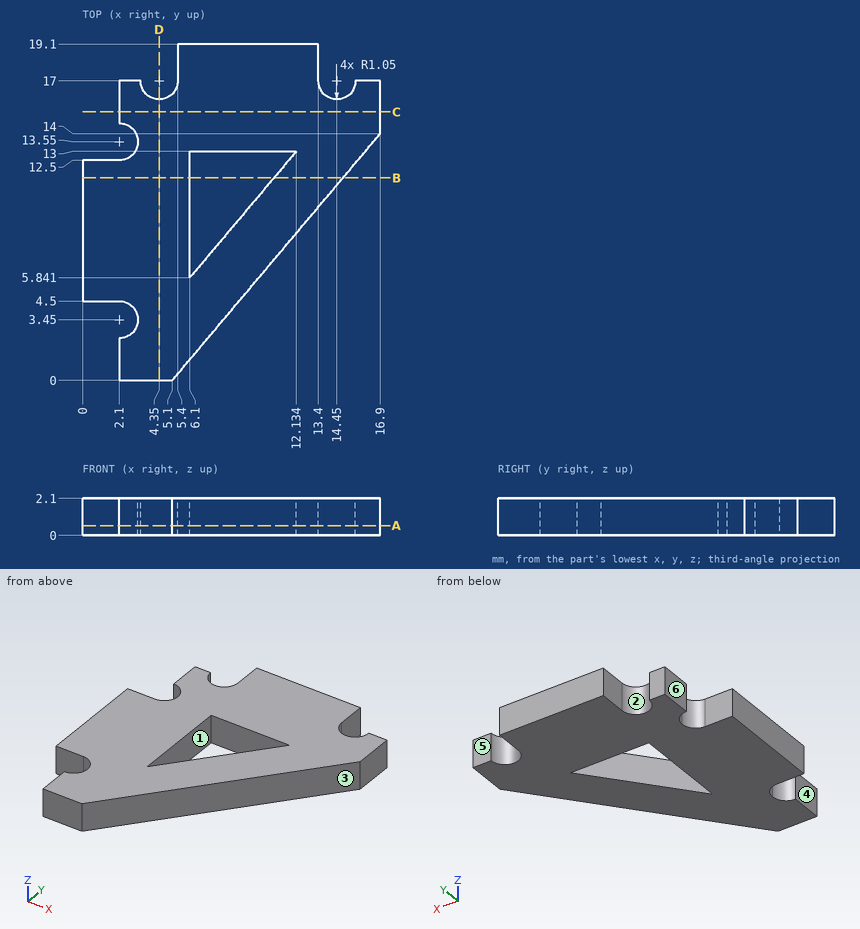
Verification items for this drawing (mm, ordinates from the low corner). A direction names the side the tool comes from. Round coordinates to 2 decimals unless told otherwise and drop trailing zeros. Order: outer loops, then holes, each group sorted by start corner. A loop starts at its lowest first (then second) coordinate and runs counter-clockwise, first axis right, second up. Notation, with made-up numbers: (-7.75, 74) - (39.25, 74) arc R10 cw to (39.25, 82) - close; hole circle Ø9 at (66, 61). An arc over 180 degrees is marked (long way). Answer as CSV lines item,"result". Start each with the question number.
1) Section check B-B (y = 11.5). Record the cut outline in (x, z).
2) Section check A-A (z = 0.55). Record the cut outline in (x, y), then the cut area to 3 significant figures.
3) Scan lines: probe 1 along Y at (x, z) = (2.5, 1.2); probe 2 along X at (y, z) = (6.75, 0.8) (1 decimal); probe 3 along X at (y, z) = (11.25, 1.9). Record each from-to range of solid material in increasing order.
4) Depth check by flat-ended pin: pin 1 (1 mm diameter, centred on y = 7, z = 0.5, fed in from +X); pin 2 (0.6 mm diameter, centred on y = 18, z = 1, fed in from +X); pin 3 (1 mm diameter, centred on y = 10.5, z = 1.5, fed in from +X). Enter the tip coordinate at first touch or a pass-through.
5) Tool access check on the marked faces 4, 5 and 6. Record the directions out of +Z, -Z, +X, -X, +Y, -Y that give a thin tool (end or side, any length) a straight path to the whole face; none if there is none.
6) Section check C-C (y = 15.25). Record the cut outline in (x, z).
7) Section check D-D (x = 4.35). Record the cut outline in (y, z), then the cut area to 3 significant figures.
8) Draft check along Y on the marked faces 1, 2 and 3. Enter one of: +Y half, -Y half, draft (parallel to the pull), parting line (faces both ways), or undercut.
Determined:
1,outline,"(0, 0) - (6.1, 0) - (6.1, 2.1) - (0, 2.1) - close; (10.87, 0) - (14.79, 0) - (14.79, 2.1) - (10.87, 2.1) - close"
2,outline,"(0, 4.5) - (2.1, 4.5) arc R1.05 cw to (2.1, 2.4) - (2.1, 0) - (5.1, 0) - (16.9, 14) - (16.9, 17) - (15.5, 17) arc R1.05 cw to (13.4, 17) - (13.4, 19.1) - (5.4, 19.1) - (5.4, 17) arc R1.05 cw to (3.3, 17) - (2.1, 17) - (2.1, 14.6) arc R1.05 cw to (2.1, 12.5) - (0, 12.5) - close; hole (6.1, 5.84) - (12.13, 13) - (6.1, 13) - close"
2,area,"174 mm^2"
3,probe 1,"0 to 2.48, 4.42 to 12.58, 14.52 to 17"
3,probe 2,"0 to 6.1, 6.9 to 10.8"
3,probe 3,"0 to 6.1, 10.66 to 14.58"
4,pin 1,"x = 11.42"
4,pin 2,"x = 13.4"
4,pin 3,"x = 14.37"
5,face 4,"+Z, -Z, -X, -Y"
5,face 5,"+Z, -Z, +X, +Y"
5,face 6,"+Z, -Z, -X, +Y"
6,outline,"(2.1, 0) - (16.9, 0) - (16.9, 2.1) - (2.1, 2.1) - close"
7,outline,"(0, 0) - (15.95, 0) - (15.95, 2.1) - (0, 2.1) - close"
7,area,"33.5 mm^2"
8,face 1,"undercut"
8,face 2,"+Y half"
8,face 3,"-Y half"
